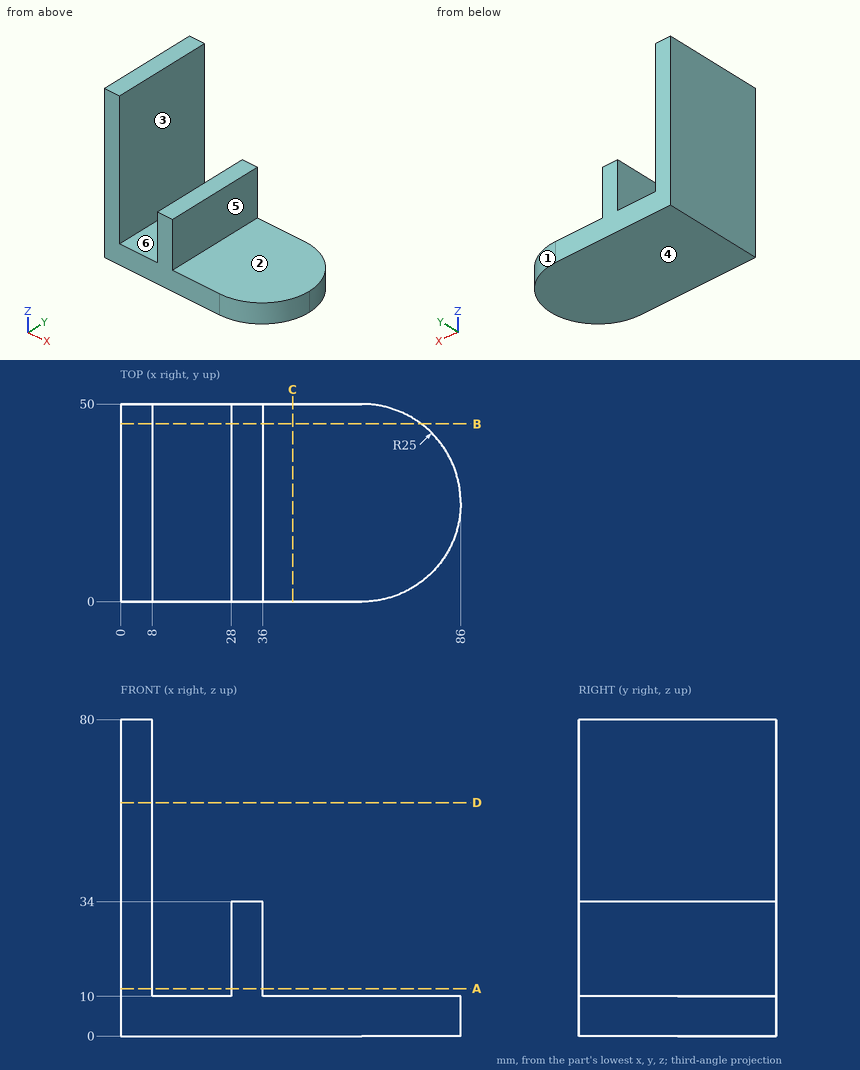
Geometry check sheet. Reference: drawing and pictorial views, mm from the part's lowest x, y, z. A direction names the side the tool comes from. Give positions to 0.01 mm unless a question says otherwise; leave off trailing zeros. Order: outer loops, then holes, each group sorted by start corner. A loop starts at its lowest first (then second) coordinate and runs counter-clockwise, first axis right, second up. Notation, with made-up numbers: M 15,65 L 73,65 A20 ccw 73,95 Z; hole C -15,23.25 d5. An arc over 180 degrees is marked long. Return JSON: item names as keys, results as strings. Group by question number.
1) Section check D-D on z = 59. Record the cut outline in (x, y), and give its area (3 significant figures).
2) Scan lines: line 1 (X direction, y = 40.5, z = 17); line 2 (Z direction, x = 41, y = 11); line 3 (X direction, y = 27.5, z = 58). Record each from-to range of solid material in increasing order.
3) Section check B-B on y = 45. Record the cut outline in (x, z).
4) Section check C-C on x = 43.5. Record the cut outline in (y, z).
5) Mould release check, pull along X, two halves, no side actions. Record for the marked faces 4, 5 and 6: pulls with the +X half, pulls with the -X half, needs draft (parallel to the pull), parting line crosses it, or undercut.
6) Section check A-A on z = 12. Record the cut outline in (x, y), and give its area (3 significant figures).
7) Access from +Z, -Z, +X, -X, +Y, -Y to the whole of each face (thin tool, end or side, straight path). Record for the marked faces 1, 2 and 3.
8) Go/stop test with flat-tipped pins: pin 1 Ø12 at (y, z) = (21, 17.5) entering from -X; pin 2 Ø16 at (x, y) = (16.5, 18.5) entering from +Z; pin 3 Ø25 at (y, z) = (24, 58) entering from +X; pin 4 Ø19 at (y, z) = (28.5, 23.5) entering from +X. Record where each tip stops, or that it passes through.
Answer block:
{
 "1": {"outline": "M 0,0 L 8,0 L 8,50 L 0,50 Z", "area": "400 mm^2"},
 "2": {"line 1": "x = 0 to 8, 28 to 36", "line 2": "z = 0 to 10", "line 3": "x = 0 to 8"},
 "3": {"outline": "M 0,0 L 76,0 L 76,10 L 36,10 L 36,34 L 28,34 L 28,10 L 8,10 L 8,80 L 0,80 Z"},
 "4": {"outline": "M 0,0 L 50,0 L 50,10 L 0,10 Z"},
 "5": {"face 4": "needs draft", "face 5": "pulls with the +X half", "face 6": "undercut"},
 "6": {"outline": "M 0,0 L 8,0 L 8,50 L 0,50 Z; M 28,0 L 36,0 L 36,50 L 28,50 Z", "area": "800 mm^2"},
 "7": {"face 1": "+Z, -Z, +X, +Y", "face 2": "+Z, +X, +Y, -Y", "face 3": "+Z, +Y, -Y"},
 "8": {"pin 1": "stops at x = 0", "pin 2": "stops at z = 10", "pin 3": "stops at x = 8", "pin 4": "stops at x = 36"}
}
